Could you check a few things on this model? Use its own coordinates, in mm. Coordinates: 2 decimals unless noted, no trailing zeros. Loops run counter-clockwise (first coordinate to the right, second up) from the corner with the lowest first, then second, coordinate; pieces in that order, holes last. Notation, with made-up numbers: (53.5, 48) -> (106.5, 48) arc R34 ccw to (106.5, 78) -> close; hole circle Ø7 at (69, -4.75). An arc over 180 degrees is marked (long way). One line per question, with ' | ' between items.
Autodesk Inventor part; units mm, degrees
ref_plane "YZ Plane" through (0, 0, 0) normal (1, 0, 0) x (0, 1, 0)
ref_plane "XZ Plane" through (0, 0, 0) normal (0, 1, 0) x (-1, 0, 0)
ref_plane "XY Plane" through (0, 0, 0) normal (0, 0, 1) x (1, 0, 0)
sketch "Sketch1" plane through (0, 0, 0) normal (0, 0, 1) x (1, 0, 0)
  line L0 (0, 0) -> (0, 120)
  circle A0 centre (80, 60) radius 50
  line L1 (0, 0) -> (150, 0)
  line L2 (150, 120) -> (0, 120)
  line L3 (0, 120) -> (0, 110)
  line L4 (0, 110) -> (5, 110)
  line L5 (5, 110) -> (5, 90)
  line L6 (5, 90) -> (0, 90)
  line L7 (0, 90) -> (0, 70)
  line L8 (0, 70) -> (5, 70)
  line L9 (5, 70) -> (5, 50)
  line L10 (5, 50) -> (0, 50)
  line L11 (0, 50) -> (0, 30)
  line L12 (0, 30) -> (5, 30)
  line L13 (5, 30) -> (5, 10)
  line L14 (5, 10) -> (0, 10)
  line L15 (0, 120) -> (-50, 120)
  line L16 (-50, 120) -> (-50, 110)
  line L17 (-50, 110) -> (-44, 110)
  line L18 (-44, 110) -> (-44, 90)
  line L19 (-44, 90) -> (-50, 90)
  line L20 (-50, 90) -> (-50, 70)
  line L21 (-50, 70) -> (-44, 70)
  line L22 (-44, 70) -> (-44, 50)
  line L23 (-44, 50) -> (-50, 50)
  line L24 (-50, 50) -> (-50, 30)
  line L25 (-50, 30) -> (-44, 30)
  line L26 (-44, 30) -> (-44, 10)
  line L27 (-44, 10) -> (-50, 10)
  line L28 (-50, 10) -> (-50, 0)
  line L29 (-50, 0) -> (0, 0)
  line L30 (150, 115) -> (145, 115)
  line L31 (145, 115) -> (145, 95)
  line L32 (150, 120) -> (200, 120)
  line L33 (200, 120) -> (200, 110)
  line L34 (200, 110) -> (194, 110)
  line L35 (194, 110) -> (194, 90)
  line L36 (194, 90) -> (200, 90)
  line L37 (200, 90) -> (200, 70)
  line L38 (200, 70) -> (194, 70)
  line L39 (194, 70) -> (194, 50)
  line L40 (194, 50) -> (200, 50)
  line L41 (200, 50) -> (200, 30)
  line L42 (200, 30) -> (194, 30)
  line L43 (194, 30) -> (194, 10)
  line L44 (194, 10) -> (200, 10)
  line L45 (200, 10) -> (200, 0)
  line L46 (200, 0) -> (150, 0)
  line L47 (150, 120) -> (150, 0)
  line L48 (145, 95) -> (150, 95)
  line L49 (150, 95) -> (150, 90)
  line L50 (150, 90) -> (145, 90)
  line L51 (145, 90) -> (145, 70)
  line L52 (145, 70) -> (150, 70)
  line L53 (0, 120) -> (0, 125)
  line L54 (150, 125) -> (150, 120)
  line L55 (0, 125) -> (10, 125)
  line L56 (10, 125) -> (10, 120)
  line L57 (10, 120) -> (30, 120)
  line L58 (30, 120) -> (30, 125)
  line L59 (30, 125) -> (50, 125)
  line L60 (50, 125) -> (50, 120)
  line L61 (50, 120) -> (70, 120)
  line L62 (70, 120) -> (70, 125)
  line L63 (70, 125) -> (90, 125)
  line L64 (90, 125) -> (90, 120)
  line L65 (90, 120) -> (110, 120)
  line L66 (110, 120) -> (110, 125)
  line L67 (110, 125) -> (130, 125)
  line L68 (130, 125) -> (130, 120)
  line L69 (130, 120) -> (140, 120)
  line L70 (140, 120) -> (140, 125)
  line L71 (140, 125) -> (150, 125)
  dimension "d12" = 100
  dimension "d13" = 120
  dimension "d14" = 150
  dimension "d17" = 80
  dimension "d18" = 60
  dimension "d19" = 10
  dimension "d20" = 5
  dimension "d21" = 20
  dimension "d22" = 20
  dimension "d23" = 5
  dimension "d24" = 20
  dimension "d25" = 20
  dimension "d26" = 20
  dimension "d38" = 50
  dimension "d39" = 10
  dimension "d40" = 6
  dimension "d41" = 5
  dimension "d42" = 5
  dimension "d43" = 50
  dimension "d44" = 6
  dimension "d45" = 5
  dimension "d46" = 20
  dimension "d47" = 20
  dimension "d48" = 5
  dimension "d51" = 10
  dimension "d52" = 20
  dimension "d53" = 20
  dimension "d54" = 20
  dimension "d55" = 20
  dimension "d56" = 20
  dimension "d57" = 20
  dimension "d58" = 10
extrude "Extrusion1" add sketch "Sketch1" against normal blind 6 contours L29 L28 L27 L26 L25 L24 L23 L22 L21 L20 L19 L18 L17 L16 L15 L0 | L0 L14 L13 L12 L10 L9 L8 L6 L5 L4 L2 L47 L30 L31 L48 L50 L51 L52 L1 | L0 L12 L13 L14 | L47 L32 L33 L34 L35 L36 L37 L38 L39 L40 L41 L42 L43 L44 L45 L46 | L52 L51 L50 L47 | L0 L8 L9 L10 | L48 L31 L30 L47 | L0 L4 L5 L6 | A0
properties part number "Archimedes Screw Border1"
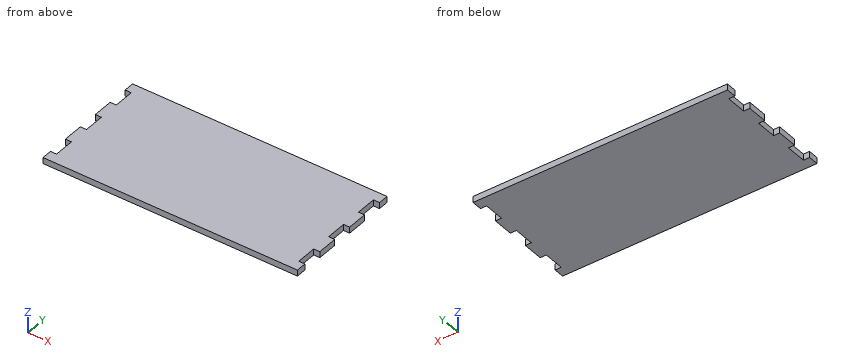
1) I'm going to push flat-ended pins straight in: pin 1 Ø3 at (y, z) = (23.5, -1.5) entering from -X; pin 2 Ø3 at (y, z) = (101, -3) entering from +X. Where does each tip first touch, or does it pass through?
Data:
pin 1: x = -44 | pin 2: x = 194
2) If we section it at B-B on y = 53: Please give me the cut outline in (x, z).
Data:
outline: (-44, -6) -> (194, -6) -> (194, 0) -> (-44, 0) -> close
3) I need wall thicknesses on line 1 along X through (y, z) = (97, -1.1). Which ranges of the line are inside material? Lowest first, please. Write a range as from..to.
Data:
line 1: -44..194
4) If we section it at A-A on z = -4.5: Please give me the cut outline in (x, y), and give its area (3 significant figures).
Data:
outline: (-50, 0) -> (200, 0) -> (200, 10) -> (194, 10) -> (194, 30) -> (200, 30) -> (200, 50) -> (194, 50) -> (194, 70) -> (200, 70) -> (200, 90) -> (194, 90) -> (194, 110) -> (200, 110) -> (200, 120) -> (-50, 120) -> (-50, 110) -> (-44, 110) -> (-44, 90) -> (-50, 90) -> (-50, 70) -> (-44, 70) -> (-44, 50) -> (-50, 50) -> (-50, 30) -> (-44, 30) -> (-44, 10) -> (-50, 10) -> close | area: 29,300 mm²
